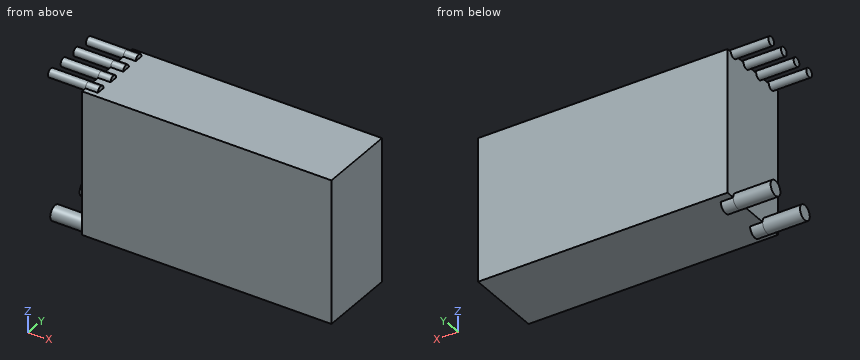
```python
from build123d import *

# Parameters (mm, degrees)
SKETCH1_W                = 50.8
SKETCH1_H                = 29.21
BOSS_EXTRUDE1_DEPTH      = 15.748
SKETCH2_R                = 1.524
SKETCH2_R_2              = 0.889
BOSS_EXTRUDE2_DEPTH      = 7.62
BOSS_EXTRUDE2_DEPTH_BACK = 2.54


with BuildPart() as part:
    # Sketch1 → Boss-Extrude1 (new body)
    with BuildSketch(Plane(origin=(0, 0, 0), x_dir=(1, 0, 0), z_dir=(0, 1, 0))):
        Rectangle(SKETCH1_W, SKETCH1_H)
    extrude(amount=BOSS_EXTRUDE1_DEPTH)

    # Sketch2 → Boss-Extrude2 (add, two sides)
    with BuildSketch(Plane.ZY.offset(25.4)) as boss_extrude2_sk:
        with Locations((-14.605, 12.446)):
            Circle(SKETCH2_R)
        with Locations((14.605, 9.8425)):
            Circle(SKETCH2_R_2)
        with Locations((14.605, 13.7795)):
            Circle(SKETCH2_R_2)
        with Locations((14.605, 5.9055)):
            Circle(SKETCH2_R_2)
        with Locations((14.605, 1.9685)):
            Circle(SKETCH2_R_2)
        with Locations((-14.605, 3.302)):
            Circle(SKETCH2_R)
    extrude(amount=BOSS_EXTRUDE2_DEPTH)
    extrude(boss_extrude2_sk.sketch, amount=-BOSS_EXTRUDE2_DEPTH_BACK)


solid = part.part
```
Part model, mm, in its own coordinate system. Round coordinates to 2 decimals unless told otherwise and drop trailing zeros. Loops run counter-clockwise (first coordinate to the right, second up) from the corner with the lowest first, then second, coordinate; pieces in that order, holes last. Notation, with made-up numbers: (57.25, 85.25) -> (112.25, 85.25) arc R18 ccw to (112.25, 94.25) -> close; hole circle Ø6 at (-5, 14.25). An arc over 180 degrees is marked (long way). Use CSV: the item, a comma, the result in double quotes. Start each with the question number.
1) Cut at A-A, the plane x = -24. Write the cut outline in (y, z) (1 decimal), plus the area to 3 significant figures.
2) Cut at C-C, the plane z = 5. Write the cut outline in (x, y).
3) Cut at B-B, the plane y = 7.5. Write the cut outline in (x, z) (3 decimals), plus the area to 3 significant figures.
4) Drop flat-ended pins along their axis: P1, Ø1.2, axis at y = 12, z = -15.5, coming from the +X side; P2, Ø6, axis at y = 12.5, z = 1.5, coming from the -X side; P3, Ø8, axis at x = 5.5, y = 7, coming from the +Z side (3 decimals). Give the stop position or say it passes through.
5) Wall check: L1, parallel to Z at x = -5, y = 1 (3 decimals); L2, parallel to X at y = 6.25, z = 6. Give the ranges that are in metal, low to high. Write a range as [from, to].
Determined:
1,outline,"(0, -14.6) -> (1.8, -14.6) arc R1.5 ccw to (4.8, -14.6) -> (10.9, -14.6) arc R1.5 ccw to (14, -14.6) -> (15.7, -14.6) -> (15.7, 14.6) -> (14.7, 14.6) arc R0.9 ccw to (12.9, 14.6) -> (10.7, 14.6) arc R0.9 ccw to (9, 14.6) -> (6.8, 14.6) arc R0.9 ccw to (5, 14.6) -> (2.9, 14.6) arc R0.9 ccw to (1.1, 14.6) -> (0, 14.6) -> close"
1,area,"472 mm2"
2,outline,"(-25.4, 0) -> (25.4, 0) -> (25.4, 15.75) -> (-25.4, 15.75) -> close"
3,outline,"(-25.4, -14.605) -> (25.4, -14.605) -> (25.4, 14.605) -> (-25.4, 14.605) -> close"
3,area,"1,480 mm2"
4,P1,"stops at x = -22.86"
4,P2,"stops at x = -25.4"
4,P3,"stops at z = 14.605"
5,L1,"z = [-14.605, 14.605]"
5,L2,"x = [-25.4, 25.4]"
